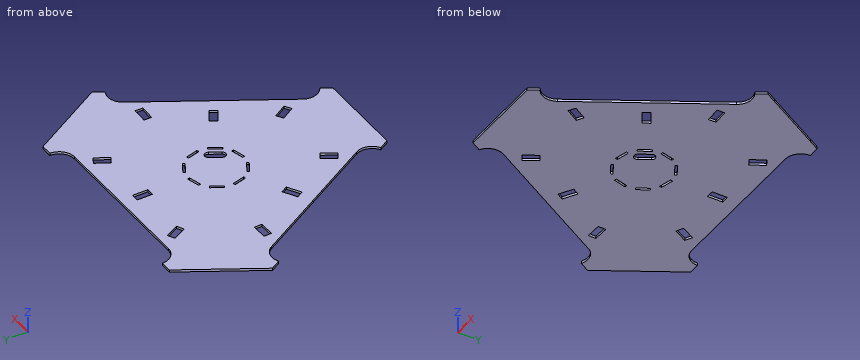
from build123d import *

# Parameters (mm, degrees)
MODEL_W                 = 10.000078668
MODEL_H                 = 19.99998508
BOSS_EXTRU_1_DEPTH      = 3
ENL_V_MAT_EXTRU_2_DEPTH = 1392.526576556


with BuildPart() as part:
    # Model → Boss.-Extru.1 (new body)
    with BuildSketch(Plane.XY):
        with BuildLine():
            Line((347.504229039, -990.984743501), (447.504154456, -1164.189847387))
            add(Edge.make_bspline(
                [(447.504154456, -1164.189847387), (453.026125757, -1173.754121475), (449.749150931, -1185.983779814), (440.184876843, -1191.505837242)],
                knots=[1, 1, 1, 1, 2, 2, 2, 2], degree=3))
            Line((440.184876843, -1191.505837242), (447.468153212, -1204.120743383))
            Line((447.468153212, -1204.120743383), (462.904937066, -1204.120743383))
            Line((462.904937066, -1204.120743383), (547.394870334, -1204.120743383))
            Line((547.394870334, -1204.120743383), (562.831654188, -1204.120743383))
            Line((562.831654188, -1204.120743383), (570.114930554, -1191.505837241))
            add(Edge.make_bspline(
                [(570.114930554, -1191.505837241), (560.550656465, -1185.983779815), (557.273681638, -1173.754121476), (562.795652937, -1164.189847387)],
                knots=[7, 7, 7, 7, 8, 8, 8, 8], degree=3))
            Line((562.795652937, -1164.189847387), (662.795578323, -990.984743483))
            add(Edge.make_bspline(
                [(662.795578323, -990.984743483), (668.317549622, -981.420469394), (680.547294088, -978.143580694), (690.111568177, -983.665465865)],
                knots=[9, 9, 9, 9, 10, 10, 10, 10], degree=3))
            Line((690.111568177, -983.665465865), (697.445659701, -970.962451406))
            Line((697.445659701, -970.962451406), (689.778082931, -957.6818667))
            Line((689.778082931, -957.6818667), (647.435103324, -884.341812722))
            Line((647.435103324, -884.341812722), (639.77820635, -871.079314757))
            Line((639.77820635, -871.079314757), (625.092281057, -871.079314757))
            add(Edge.make_bspline(
                [(625.092281057, -871.079314757), (625.092281058, -882.124979905), (616.137961126, -891.079299838), (605.092295979, -891.079299839)],
                knots=[17, 17, 17, 17, 18, 18, 18, 18], degree=3))
            Line((605.092295979, -891.079299839), (405.092272921, -891.079299839))
            add(Edge.make_bspline(
                [(405.092272921, -891.079299839), (394.046607773, -891.07929984), (385.09228784, -882.124979908), (385.092287839, -871.079314761)],
                knots=[19, 19, 19, 19, 20, 20, 20, 20], degree=3))
            Line((385.092287839, -871.079314761), (370.370533553, -871.079314761))
            Line((370.370533553, -871.079314761), (312.778700066, -970.831623929))
            Line((312.778700066, -970.831623929), (320.188239184, -983.665465888))
            add(Edge.make_bspline(
                [(320.188239184, -983.665465888), (329.752513272, -978.143494587), (341.982257738, -981.420469413), (347.504229039, -990.984743501)],
                knots=[23, 23, 23, 23, 24, 24, 24, 24], degree=3))
        make_face()
        Polygon((622.618702509, -993.05007822), (642.608524558, -993.687248628), (642.290025481, -1003.682159653), (622.300031178, -1003.044989244), align=None, mode=Mode.SUBTRACT)
        Polygon((594.878104643, -1072.794736968), (577.611630575, -1062.701812979), (582.658178697, -1054.068575945), (599.924652765, -1064.161499934), align=None, mode=Mode.SUBTRACT)
        Polygon((583.685161648, -902.731560157), (592.474806017, -907.50051971), (582.937059165, -925.079722321), (574.147414796, -920.310848895), align=None, mode=Mode.SUBTRACT)
        Polygon((552.326007751, -1122.752411126), (562.689371739, -1139.857999232), (554.136577686, -1145.039681226), (543.773213697, -1127.93409312), align=None, mode=Mode.SUBTRACT)
        with Locations((505.092198326, -918.785791257)):
            Rectangle(MODEL_W, MODEL_H, mode=Mode.SUBTRACT)
        Polygon((458.493147779, -1123.193383356), (467.045941833, -1128.375065349), (456.682577848, -1145.480653457), (448.129783794, -1140.298971465), align=None, mode=Mode.SUBTRACT)
        Polygon((425.950948052, -902.731560171), (435.488694907, -920.310848907), (426.699050539, -925.079722335), (417.161303684, -907.500519726), align=None, mode=Mode.SUBTRACT)
        Polygon((428.161149075, -1054.509548181), (433.207697199, -1063.142785214), (415.941223133, -1073.235709206), (410.894675009, -1064.602472173), align=None, mode=Mode.SUBTRACT)
        Polygon((388.200625252, -993.491050463), (388.519124331, -1003.485961487), (368.529302282, -1004.123131899), (368.210803204, -994.128220875), align=None, mode=Mode.SUBTRACT)
    extrude(amount=BOSS_EXTRU_1_DEPTH)

    # Esquisse2 → Enlèv. mat.-Extru.2 (cut, through all)
    with BuildSketch(Plane(origin=(0, 0, 0), x_dir=(-1, 0, 0), z_dir=(0, 0, -1))):
        with BuildLine():
            Line((-526.434334105, -1036.035042627), (-533.934329365, -1023.044658352))
            add(Edge.make_bspline(
                [(-533.934329365, -1023.044658352), (-535.315042909, -1020.653190239), (-534.495664502, -1017.595243477), (-532.104199693, -1016.21453184)],
                knots=[1, 1, 1, 1, 2, 2, 2, 2], degree=3))
            add(Edge.make_bspline(
                [(-532.104199693, -1016.21453184), (-529.712734884, -1014.833820204), (-526.654786726, -1015.653193399), (-525.274073182, -1018.044661512)],
                knots=[2, 2, 2, 2, 3, 3, 3, 3], degree=3))
            Line((-525.274073182, -1018.044661512), (-517.774077922, -1031.035045787))
            add(Edge.make_bspline(
                [(-517.774077922, -1031.035045787), (-516.393364378, -1033.4265139), (-517.212742785, -1036.484460663), (-519.604207594, -1037.865172299)],
                knots=[4, 4, 4, 4, 5, 5, 5, 5], degree=3))
            add(Edge.make_bspline(
                [(-519.604207594, -1037.865172299), (-521.995672403, -1039.245883936), (-525.053620562, -1038.42651074), (-526.434334105, -1036.035042627)],
                knots=[5, 5, 5, 5, 6, 6, 6, 6], degree=3))
        make_face()
        Polygon((-466.912163294, -1016.838076711), (-471.311987833, -1033.258962352), (-474.209588183, -1032.482769314), (-469.809499355, -1016.061731085), align=None)
        Polygon((-505.784176347, -1050.63498378), (-522.204989382, -1046.234888271), (-522.981588875, -1049.132379712), (-506.560775841, -1053.532475221), align=None)
        Polygon((-543.414554373, -1013.888013101), (-540.516954023, -1014.664206139), (-536.117129484, -998.243320497), (-539.014729835, -997.467127459), align=None)
        Polygon((-487.287063031, -981.399673764), (-503.708140356, -976.999730842), (-504.48424394, -979.898081226), (-488.064270392, -984.297516156), align=None)
        Polygon((-539.08988115, -1025.104375563), (-530.589886522, -1039.826811075), (-533.187963377, -1041.326810127), (-541.687958005, -1026.604374615), align=None)
        Polygon((-516.425728308, -978.663411899), (-514.925729256, -981.261488754), (-529.648164768, -989.761483382), (-531.14816382, -987.163406527), align=None)
        Polygon((-479.095212457, -1043.319423279), (-480.595215323, -1040.721339817), (-495.317650835, -1049.221334445), (-493.817647969, -1051.819417907), align=None)
        Polygon((-476.996433275, -989.335575737), (-468.496438647, -1004.058011249), (-471.094515502, -1005.558010301), (-479.59451013, -990.835574789), align=None)
    extrude(amount=-ENL_V_MAT_EXTRU_2_DEPTH, mode=Mode.SUBTRACT)


solid = part.part
CAD build for the part. Positions are in the model's coordinates, mm. Round coordinates to 2 decimals unless told otherwise and drop trailing zeros. Write each loop counter-clockwise with the first axis right and the second up, starting at its lowest first coordinate (ties: lowest second). Pieces come first, ordered by that corner, then holes.
(1) Slice it at B-B, the plane y = -936.5. Write the cut outline in (x, z).
(2) Slice it at C-C, the plane y = -1091.5. Write the cut outline in (x, z).
(3) Slice it at A-A, the plane z = 1.9. Count the separate pieces of the cut face and the enclosed holes in it, and give its area (3 significant figures).
(4) Probe line 1 along Y through (x, z) = (508, 0.7); line 2 along Y through (x, z) = (479, 0.7); line 3 along X through (y, z) = (-1064, 1.7). List the from-to ranges inside material, lowest first.
(5) Drop flat-ended pins along their axis: P1, Ø0.9, axis at y = -921.5, z = 1, coming from the -X side; P2, Ø6, axis at x = 475, y = -951.5, coming from the -Z side; P3, Ø1.5, axis at y = -918.5, z = 1, coming from the +X side; P4, Ø0.9, axis at x = 522, z = 1.5, coming from the +Y side. Give the stop position or say it passes through.
From the geometry:
1. outline: (332.6, 0) - (677.55, 0) - (677.55, 3) - (332.6, 3) - close
2. outline: (405.54, 0) - (604.76, 0) - (604.76, 3) - (405.54, 3) - close
3. separate pieces: 1
3. enclosed holes: 18
3. area: 74,600 mm2
4. line 1: y = -1204.12 to -1053.15, -1050.04 to -928.79, -908.79 to -891.08
4. line 2: y = -1204.12 to -991.87, -990.49 to -891.08
4. line 3: x = 389.66 to 411.93, 431.74 to 579.83, 599.65 to 620.64
5. P1: stops at x = 341
5. P2: stops at z = 0
5. P3: stops at x = 667.59
5. P4: stops at y = -891.08
